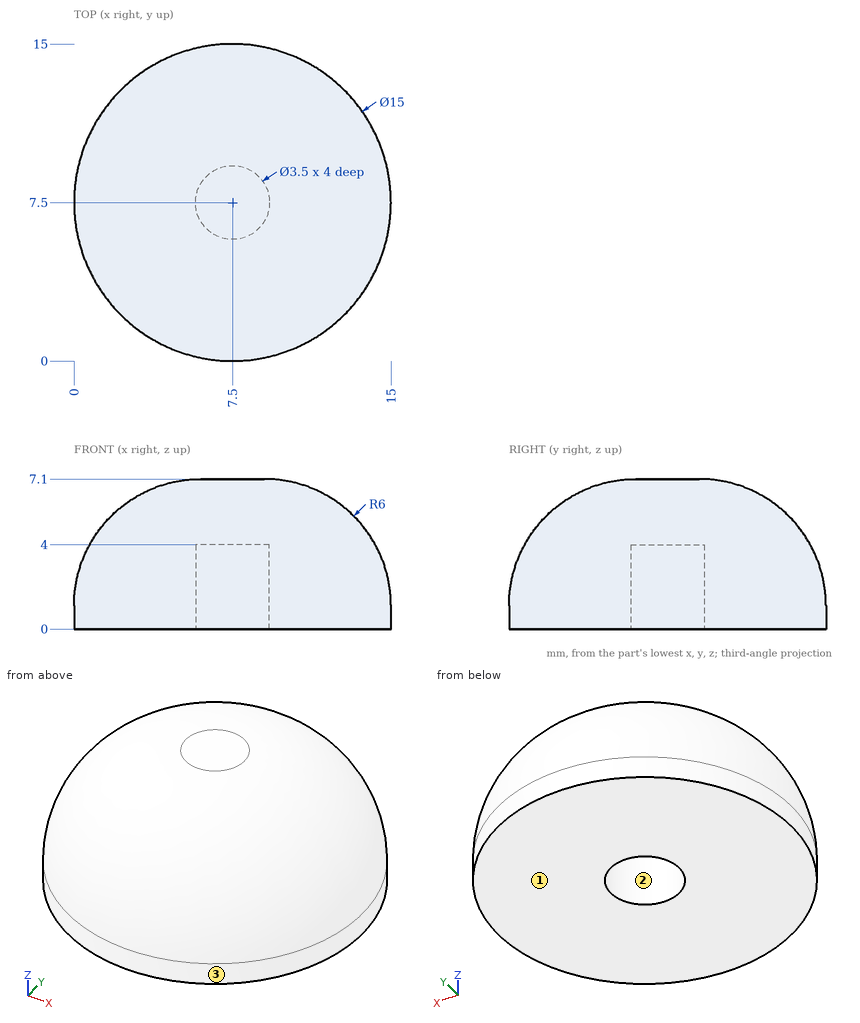
Job drawing, mm, ordinate dimensions from the low corner. One solid piece. Give positions to 0.01 mm unless a question says otherwise; leave off trailing zeros. Return JSON: item names as keys, results as strings.
1) Probe line 1 (Y direction, x = 7.5, z = 1); line 2 (X direction, y = 6.5, z = 3); line 3 (Z direction, x = 7.25, y = 14.25). List the from-to ranges inside material, lowest first. Write a range as from..to.
Geometry says:
{"line 1": "0..5.75, 9.25..15", "line 2": "0.38..6.06, 8.94..14.62", "line 3": "0..4"}
2) Pull direction X, two halves, no side cores. Call the marked faces 1, 2 and 3: pulls with the +X half, pulls with the -X half, needs draft (parallel to the pull), parting line crosses it, or undercut.
Geometry says:
{"face 1": "needs draft", "face 2": "undercut", "face 3": "parting line crosses it"}
3) Flat gauge pins, fed straight in: P1, Ø3, axis at x = 2, z = 3, coming from the -Y side; P2, Ø4, axis at y = 4, z = 4.5, coming from the -X side; P3, Ø4, axis at x = 3.5, z = 4, coming from the -Y side. Where does each tip first touch, or does it go through?
Geometry says:
{"P1": "y = 1.41", "P2": "x = 0.65", "P3": "y = 0.65"}
